```python
from build123d import *

# Parameters (mm, degrees)
REVOLUTION_ANGLE = 180
PAD_DEPTH        = 60
SKETCH002_R      = 3
HOLE_DEPTH       = 131.001


with BuildPart() as part:
    # Sketch → Revolution (revolve)
    with BuildSketch(Plane.XZ):
        with BuildLine():
            ThreePointArc((117, 0), (0, 117), (-117, 0))
            Line((-117, 0), (-113, 0))
            ThreePointArc((113, 0), (0, 113), (-113, 0))
            Line((113, 0), (117, 0))
        make_face()
    revolve(axis=Axis((0, 0, 0), (1, 0, 0)), revolution_arc=REVOLUTION_ANGLE)

    # Sketch001 → Pad (new body)
    with BuildSketch(Plane.XZ):
        Polygon((-100, 14), (-100, -14), (-135, -14), (-135, -10), (-122, -10), (-122, 10), (-135, 10), (-135, 14), align=None)
    extrude(amount=PAD_DEPTH)

    # Sketch002 (on Face3 of Pad) → Hole (cut, through all)
    with BuildSketch(Plane(origin=(0, 0, 14), x_dir=(-1, 0, 0), z_dir=(0, 0, 1))):
        with Locations((128.5, 10)):
            Circle(SKETCH002_R)
        with Locations((128.5, 30)):
            Circle(SKETCH002_R)
        with Locations((128.5, 50)):
            Circle(SKETCH002_R)
    extrude(amount=-HOLE_DEPTH, mode=Mode.SUBTRACT)


solid = part.part
```
The listing builds one solid part. Answer for the finished solid, in the listing's coordinates (mm). A direction names the side the tool comes from. Give positions to 0.01 mm unless a question says otherwise; leave off trailing zeros. Write each loop counter-clockwise with the first axis right and the second up, starting at its lowest first coordinate (ties: lowest second). Pieces come first, ordered by that corner, then holes. Notation, with made-up numbers: (0.25, 86.25) -> (54.25, 86.25) arc R14 cw to (54.25, 103.25) -> close; hole circle Ø10 at (20, -7.5). An arc over 180 degrees is marked (long way). Write item = value, one per line. Start each with the question number.
1) The part is cut by section A-A, the plane x = -128.5. Count the separate pieces of the cut face and the enclosed holes in it, and give its area (3 significant figures).
2) Determine the mould class of faces 4 (the face through (-131.36, -50.9, 12.03)), 5 (the face through (-133, -30, -10)), 6 (the face through (-102, 0, 9)) for opening direction Y: +Y half, -Y half, draft (parallel to the pull), parting line (faces both ways), or undercut.
3) The part is cut by section B-B, the plane y = -10. Determine the outline of the cut face in (x, z), and give its area (3 significant figures).
4) Straight lines are drawn through the part: line 1 along Y through (x, z) = (-128.5, -12.35); line 2 along X through (y, z) = (-30, 11); line 3 along X through (y, z) = (-50, -12.85). For each, find the intervals that lie inside material, in ascending order.
5) Which of the six approach directions +Z, -Z, +X, -X, +Y, -Y give full straight-line access (tool end or side, diameter ignored) to faces 1 (the face through (-124, -30, 10)), 2 (the face through (-100, -26, 0)), 3 (the face through (-121, -36, -14))?
6) Each of these flat-tipped pins is pushed along its axis until it touches: pin 1 (3.5 mm diameter, centred on x = -128.5, y = -50, fed in from +Z); pin 2 (14.5 mm diameter, centred on x = -128, y = -27.5, fed in from +Z); pin 3 (3 mm diameter, centred on y = -84, z = 47, fed in from -X); pin 4 (1.5 mm diameter, centred on y = -13.5, z = 90.5, fed in from +X). Where does it stop, or does it pass through?
7) The part is cut by section D-D, the plane x = -51. Determine the outline of the cut face in (y, z), and give its area (3 significant figures).
8) The part is cut by section C-C, the plane y = -30. Determine the outline of the cut face in (x, z), and give its area (3 significant figures).
Solutions:
q1.separate_pieces = 8
q1.enclosed_holes = 0
q1.area = 336 mm²
q2.face_4 = undercut
q2.face_5 = draft
q2.face_6 = +Y half
q3.outline = (-135, -14) -> (-131.5, -14) -> (-131.5, -10) -> (-135, -10) -> close; (-135, 10) -> (-131.5, 10) -> (-131.5, 14) -> (-135, 14) -> close; (-125.5, -14) -> (-115.73, -14) arc R116.57 ccw (long way) to (-115.73, 14) -> (-125.5, 14) -> (-125.5, 10) -> (-122, 10) -> (-122, -10) -> (-125.5, -10) -> close; hole (-111.68, -14) arc R112.56 ccw (long way) to (-111.68, 14) -> (-100, 14) -> (-100, -14) -> close
q3.area = 3,450 mm²
q4.line_1 = -60 to -53, -47 to -33, -27 to -13, -7 to 0
q4.line_2 = -135 to -131.5, -125.5 to -100, 108.39 to 112.55
q4.line_3 = -135 to -131.5, -125.5 to -100, 100.52 to 104.99
q5.face_1 = -X, +Y, -Y
q5.face_2 = +Y
q5.face_3 = -Z, -X, -Y
q6.pin_1 = through
q6.pin_2 = 14
q6.pin_3 = -68.63
q6.pin_4 = 73.85
q7.outline = (0, -105.3) -> (0, -100.84) arc R100.84 cw to (0, 100.84) -> (0, 105.3) arc R105.3 ccw to start
q7.area = 1,450 mm²
q8.outline = (-135, -14) -> (-131.5, -14) -> (-131.5, -10) -> (-135, -10) -> close; (-135, 10) -> (-131.5, 10) -> (-131.5, 14) -> (-135, 14) -> close; (-125.5, -14) -> (-112.22, -14) arc R113.09 ccw (long way) to (-112.22, 14) -> (-125.5, 14) -> (-125.5, 10) -> (-122, 10) -> (-122, -10) -> (-125.5, -10) -> close; hole (-108.04, -14) arc R108.94 ccw (long way) to (-108.04, 14) -> (-100, 14) -> (-100, -14) -> close
q8.area = 3,450 mm²
